The model under review builds one solid part; all positions refer to its coordinate system, in mm. A direction names the side the tool comes from. Give positions to 0.01 mm unless a question says otherwise; leave off trailing zeros. Write each loop counter-clockwise with the first axis right and the second up, starting at its lowest first coordinate (ties: lowest second). Pieces come first, ordered by that corner, then holes.
from build123d import *

# Parameters (mm, degrees)
F0_W     = 26
F0_H     = 17
F1_DEPTH = 3
F2_W     = 13
F2_H     = 2.75
F3_DEPTH = 4
F7_DEPTH = 4.5
F8_W     = 3.3
F8_H     = 20.4774261328
F9_DEPTH = 25
F10_R    = 1


with BuildPart() as f1:
    # F0 (on Top) → F1 (new body)
    with BuildSketch(Plane.XY):
        with Locations((13, 8.5)):
            Rectangle(F0_W, F0_H)
    extrude(amount=F1_DEPTH)

    # F2 (on face) → F3 (join)
    with BuildSketch(Plane.XY.offset(3)):
        Polygon((26, 0), (26, 9.75), (23.25, 9.75), (23.25, 2.75), (18.25, 2.75), (18.25, 0), align=None)
        with Locations((16.75, 15.625)):
            Rectangle(F2_W, F2_H)
        Polygon((2.75, 17), (0, 17), (0, 0), (7.75, 0), (7.75, 2.75), (2.75, 2.75), align=None)
    extrude(amount=F3_DEPTH)

    # F6 (on plane+point) → F7 (join, symmetric)
    with BuildSketch(Plane(origin=(13, 0, 0), x_dir=(0, -1, 0), z_dir=(-1, 0, 0))):
        with BuildLine():
            Line((0, -10), (0, 0))
            Line((0, 0), (-17, 0))
            Line((-17, 0), (-17, -10))
            ThreePointArc((-17, -10), (-8.5, -1.5), (0, -10))
        make_face()
        with BuildLine():
            ThreePointArc((-17, -10), (-8.5, -18.5), (0, -10))
            Line((0, -10), (-5.75, -10))
            ThreePointArc((-5.75, -10), (-8.5, -12.75), (-11.25, -10))
            Line((-11.25, -10), (-17, -10))
        make_face()
        with BuildLine():
            Line((-5.75, -10), (0, -10))
            ThreePointArc((0, -10), (-8.5, -1.5), (-17, -10))
            Line((-17, -10), (-11.25, -10))
            ThreePointArc((-11.25, -10), (-8.5, -7.25), (-5.75, -10))
        make_face()
    extrude(amount=F7_DEPTH, both=True)

    # F8 (on face) → F9 (cut)
    with BuildSketch(Plane(origin=(0, 17, 0), x_dir=(-1, 0, 0), z_dir=(0, 1, 0))):
        with Locations((-13, -10.2387130664)):
            Rectangle(F8_W, F8_H)
    extrude(amount=-F9_DEPTH, mode=Mode.SUBTRACT)

    # F10
    f10_edges = [f1.edges().sort_by_distance(p)[0] for p in [
        (20.75, 2.75, 3),
        (5.25, 2.75, 3),
        (8.5, 8.5, 0),
        (17.5, 8.5, 0),
        (14.65, 8.5, 0),
        (11.35, 8.5, 0),
    ]]
    fillet(f10_edges, radius=F10_R)


solid = f1.part
1) The part is to be moulded in two halves that separate along X. For faces 1 (the cylindrical face through (5.215, 3.051, 3.285)), 2 (the flat face through (8.5, 6.7, -7.7)), 3 (the cylindrical face through (9.91, 7.02, -12.32)), say which applies: +X half, -X half, draft (parallel to the pull), parting line (faces both ways), or undercut.
2) Consider section D-D, the plane y = 12.5. Give the boundary of the cut face in (x, z).
3) To check wall thickness, follow probe 1 along Z at (x, y) = (10.2, 8.5); probe 2 along X at (y, z) = (9, -1.25); probe 3 along Y at (x, z) = (19.25, 6). State the ranges of each line that lie inside material, in increasing order.
4) Consider section A-A, the plane y = 8.5. Give the boundary of the cut face in (x, z), then the cut area to 3 significant figures.
5) Consider section C-C, the plane z = -3. Give the boundary of the cut face in (x, y), then the cut area to 3 significant figures.
6) Tool access review of faces 4 (the flat face through (18.25, 1, 5)), 5 (the flat face through (10.25, 16, 5)), 6 (the cylindrical face through (14.349, 8.381, -0.285)), 7 (the flat face through (23.25, 16, 5)), 8 (the flat face through (21, 2.75, 5)): name each direction out of +Z, -Z, +X, -X, +Y, -Y from which nothing blocks a thin tool from reaching the whole face with its end or side.
7) Insertion check: pin 1 (2 mm diameter, centred on x = 4.5, y = 9.5, fed in from -Z); pin 2 (5 mm diameter, centred on x = 9.5, y = 11.5, fed in from +Z); pin 3 (7 mm diameter, centred on y = 8.5, z = -10, fed in from -X). Each pin has a flat end and moves straight along its axis. Give the tip position at first contact, or say it passes through.
8) Consider section B-B, the plane x = 16.25. Give the boundary of the cut face in (y, z), then the cut area to 3 significant figures.
Answer block:
1. face 1: undercut
1. face 2: -X half
1. face 3: draft
2. outline: (0, 0) - (7.5, 0) arc R1 cw to (8.5, -1) - (8.5, -17.5) - (11.35, -17.5) - (11.35, -1) arc R1 cw to (12.35, 0) - (13.65, 0) arc R1 cw to (14.65, -1) - (14.65, -17.5) - (17.5, -17.5) - (17.5, -1) arc R1 cw to (18.5, 0) - (26, 0) - (26, 3) - (2.75, 3) - (2.75, 7) - (0, 7) - close
3. probe 1: z = -18.5 to -12.75, -7.25 to 3
3. probe 2: x = 8.5 to 11.35, 14.65 to 17.5
3. probe 3: y = 0 to 2.75, 14.25 to 17
4. outline: (0, 0) - (7.5, 0) arc R1 cw to (8.5, -1) - (8.5, -7.25) - (11.35, -7.25) - (11.35, -1) arc R1 cw to (12.35, 0) - (13.65, 0) arc R1 cw to (14.65, -1) - (14.65, -7.25) - (17.5, -7.25) - (17.5, -1) arc R1 cw to (18.5, 0) - (26, 0) - (26, 7) - (23.25, 7) - (23.25, 3) - (2.75, 3) - (2.75, 7) - (0, 7) - close; (8.5, -18.5) - (11.35, -18.5) - (11.35, -12.75) - (8.5, -12.75) - close; (14.65, -18.5) - (17.5, -18.5) - (17.5, -12.75) - (14.65, -12.75) - close
4. area: 175 mm2
5. outline: (8.5, 0) - (11.35, 0) - (11.35, 17) - (8.5, 17) - close; (14.65, 0) - (17.5, 0) - (17.5, 17) - (14.65, 17) - close
5. area: 96.9 mm2
6. face 4: +Z, -Y
6. face 5: +Z, +Y, -Y
6. face 6: -Z, +Y, -Y
6. face 7: +Z, +X, +Y
6. face 8: +Z
7. pin 1: stops at z = 0
7. pin 2: stops at z = 3
7. pin 3: stops at x = 8.5
8. outline: (0, -10) arc R8.5 ccw to (17, -10) - (17, 7) - (14.25, 7) - (14.25, 3) - (0, 3) - close; hole circle Ø5.5 at (8.5, -10)
8. area: 322 mm2
